Here's the drawing with two shaded views (mm, measured from the low corner). I have some questions. A direction names the side the tool comes from. Round coordinates to 2 decimals unless told otherwise and drop trailing zeros. Write each loop counter-clockwise with the first axis right and the second up, starting at its lowest first coordinate (ties: lowest second). Pieces come first, ordered by that corner, then holes. Notation, with made-up numbers: (17, 38) - (64, 38) arc R31 ccw to (64, 69) - close; hole circle Ø2 at (4.25, 37). An arc over 180 degrees is marked (long way). Return JSON: item names as keys, results as strings. Group by question number.
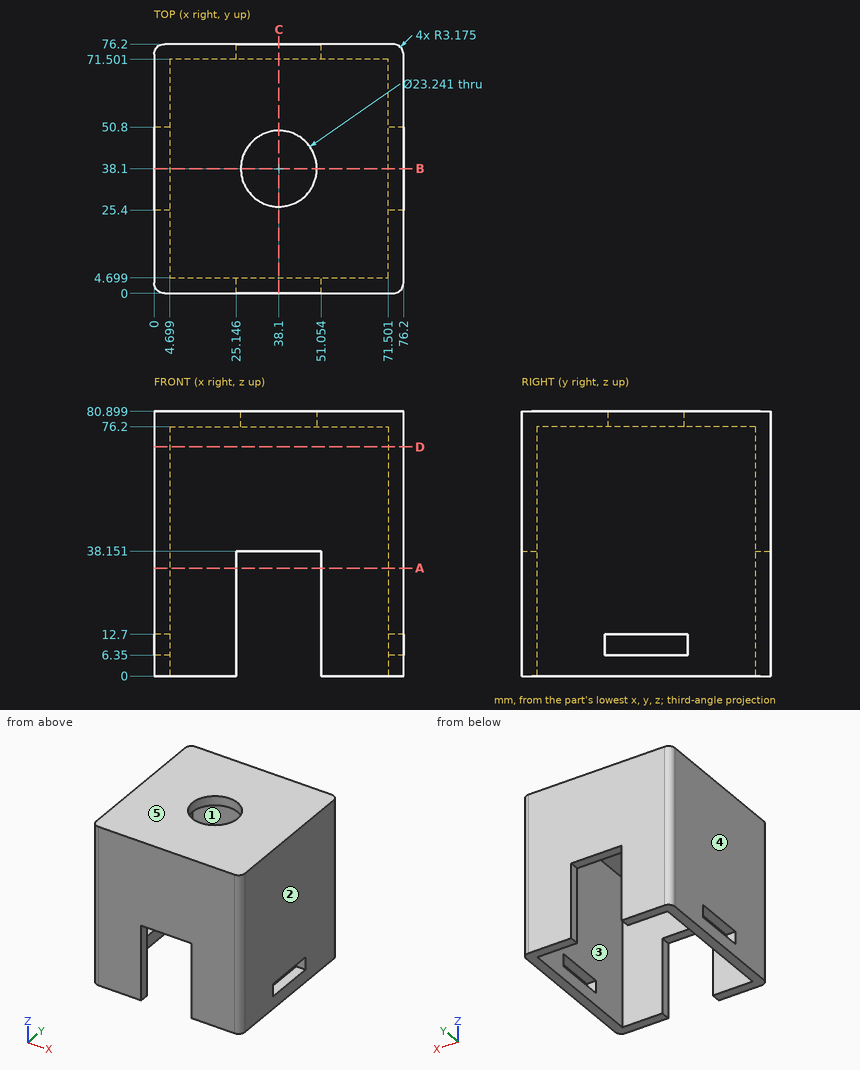
1) Imagine slicing it at B-B (y = 38.1). Please give me the cut outline in (x, z), plus the area to 3 significant figures.
2) Imagine slicing it at C-C (x = 38.1). Please give me the cut outline in (y, z).
3) Imagine slicing it at A-A (z = 33). Please give me the cut outline in (x, y) (3 decimals), plus the area to 3 significant figures.
4) For the marked faces 1 and 2, which set-ups out of +Z, -Z, +X, -X, +Y, -Y let a thin tool reach every point of the face, with its end or its side?
5) Will these pins go through, and if not, where does the flat tip stop? pin 1 Ø5 at (x, z) = (11, 63.5) entering from -Y; pin 2 Ø1.4 at (x, y) = (37, 75) entering from -Z; pin 3 Ø1.4 at (y, z) = (2, 28) entering from +X.
6) If we mould it in two halves opening along X, with no side actions, what happens to the marked faces 3, 4 and 5? For each: released by +X, released by -X, zero draft, split by the parting line, or undercut.
7) Imagine slicing it at D-D (z = 70). Please give me the cut outline in (x, y) (3 decimals).
8) I need wall thicknesses on line 1 along X through (y, z) = (29.5, 50); line 2 along Y through (x, z) = (38, 78). Which ranges of each line are inside material? Lowest first, please.
Results found:
{
 "1": {"outline": "(0, 0) - (4.7, 0) - (4.7, 6.35) - (0, 6.35) - close; (0, 12.7) - (4.7, 12.7) - (4.7, 76.2) - (26.48, 76.2) - (26.48, 80.9) - (0, 80.9) - close; (49.72, 76.2) - (71.5, 76.2) - (71.5, 12.7) - (76.2, 12.7) - (76.2, 80.9) - (49.72, 80.9) - close; (71.5, 0) - (76.2, 0) - (76.2, 6.35) - (71.5, 6.35) - close", "area": "905 mm²"},
 "2": {"outline": "(0, 38.15) - (4.7, 38.15) - (4.7, 76.2) - (26.48, 76.2) - (26.48, 80.9) - (0, 80.9) - close; (49.72, 76.2) - (71.5, 76.2) - (71.5, 38.15) - (76.2, 38.15) - (76.2, 80.9) - (49.72, 80.9) - close"},
 "3": {"outline": "(0, 3.175) arc R3.175 ccw to (3.175, 0) - (25.146, 0) - (25.146, 4.699) - (4.699, 4.699) - (4.699, 71.501) - (25.146, 71.501) - (25.146, 76.2) - (3.175, 76.2) arc R3.175 ccw to (0, 73.025) - close; (51.054, 0) - (73.025, 0) arc R3.175 ccw to (76.2, 3.175) - (76.2, 73.025) arc R3.175 ccw to (73.025, 76.2) - (51.054, 76.2) - (51.054, 71.501) - (71.501, 71.501) - (71.501, 4.699) - (51.054, 4.699) - close", "area": "1,090 mm²"},
 "4": {"face 1": "-Z", "face 2": "+Z, -Z, +X, +Y, -Y"},
 "5": {"pin 1": "stops at y = 0", "pin 2": "stops at z = 38.15", "pin 3": "stops at x = 76.16"},
 "6": {"face 3": "undercut", "face 4": "released by -X", "face 5": "zero draft"},
 "7": {"outline": "(0, 3.175) arc R3.175 ccw to (3.175, 0) - (73.025, 0) arc R3.175 ccw to (76.2, 3.175) - (76.2, 73.025) arc R3.175 ccw to (73.025, 76.2) - (3.175, 76.2) arc R3.175 ccw to (0, 73.025) - close; hole (4.699, 4.699) - (71.501, 4.699) - (71.501, 71.501) - (4.699, 71.501) - close"},
 "8": {"line 1": "x = 0 to 4.7, 71.5 to 76.2", "line 2": "y = 0 to 26.48, 49.72 to 76.2"}
}
